from build123d import *

# Parameters (mm, degrees)
EXTRUDE_1_DEPTH     = 10
SKETCH_2_R          = 1.5
CUT_EXTRUDE_1_DEPTH = 10
CUT_EXTRUDE_2_REACH = 25.452
SKETCH_3_R          = 2


with BuildPart() as part:
    # 草图1 → 凸台-拉伸1 (new, symmetric)
    with BuildSketch(Plane.XY):
        Polygon((7.5, 0), (-7.5, 0), (-7.5, 15), (-15, 15), (-15, -5), (15, -5), (15, 15), (7.5, 15), align=None)
    extrude(amount=EXTRUDE_1_DEPTH, both=True)

    # 草图2 → 切除-拉伸1 (cut)
    with BuildSketch(Plane(origin=(0, 15, 0), x_dir=(1, 0, 0), z_dir=(0, 1, 0))):
        with Locations(Location((-11.1, 5, 0), (0, 0, 180))):
            Circle(SKETCH_2_R)
        with Locations(Location((11.1, -5, 0), (0, 0, 180))):
            Circle(SKETCH_2_R)
        with Locations((11.1, 5)):
            Circle(SKETCH_2_R)
        with Locations((-11.1, -5)):
            Circle(SKETCH_2_R)
    extrude(amount=-CUT_EXTRUDE_1_DEPTH, mode=Mode.SUBTRACT)

    # 草图3 → 切除-拉伸2 (cut, up to next)
    with BuildSketch(Plane(origin=(0, 0, 0), x_dir=(1, 0, 0), z_dir=(0, 1, 0)), mode=Mode.PRIVATE) as cut_extrude_2_sk1:
        with Locations(Location((0, 0, 0), (0, 0, 180))):
            Circle(SKETCH_3_R)
    cut_extrude_2_tool1 = extrude(cut_extrude_2_sk1.sketch, amount=-CUT_EXTRUDE_2_REACH, mode=Mode.PRIVATE) & part.part
    add(cut_extrude_2_tool1.solids().sort_by_distance((0, 0, 0))[0], mode=Mode.SUBTRACT)


solid = part.part
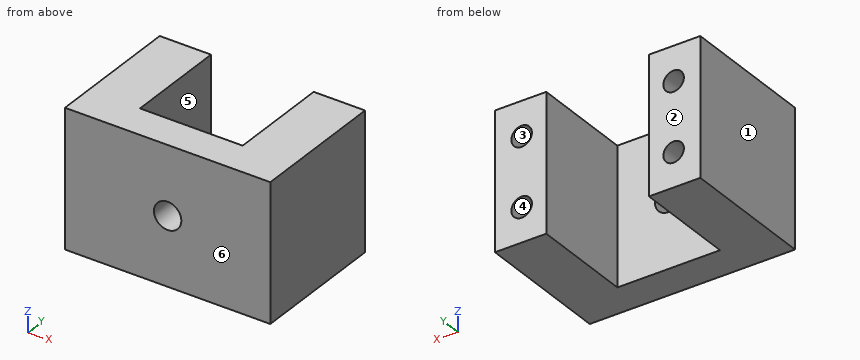
Work out the finished part from the listing and answer in its coordinate system (mm). Face numbers are marked on the shaded views. A direction names the side the tool comes from. Round coordinates to 2 decimals unless told otherwise and drop trailing zeros. Loops run counter-clockwise (first coordinate to the right, second up) from the corner with the lowest first, then second, coordinate; pieces in that order, holes last. Notation, with made-up numbers: (14.25, -35.75) - (27.25, -35.75) arc R32 ccw to (27.25, -9.75) - close; hole circle Ø6 at (60.25, 66.25). An arc over 180 degrees is marked (long way). Use one line per item in the form item = value. Start each with the question number.
(1) Find section A-A on y = 6.25. Determine the outline of the cut face in (x, z), and give its area (3 significant figures).
(2) Consider line 1 (Z direction, x = -11.1, y = 8.25); line 2 (Z direction, x = 0, y = -2.2); line 3 (X direction, y = 6.5, z = 2). Determine where each line is inside the solid, lowest interval first.
(3) Find section D-D on z = 5. Determine the outline of the cut face in (x, y), and give its area (3 significant figures).
(4) Determine the mould class of the marked faces 1, 2 and 3 for opening direction X: +X half, -X half, draft (parallel to the pull), parting line (faces both ways), or undercut.
(5) Find section C-C on x = 0. Determine the outline of the cut face in (y, z), and give its area (3 significant figures).
(6) Which of the six approach directions +Z, -Z, +X, -X, +Y, -Y give full straight-line access (tool end or side, diameter ignored) to the marked faces 4, 5 and 6?
(7) Flat-ended cylindrical pins translate along their axes: P1, Ø1.5, axis at x = 10.5, z = -5, coming from the +Y side; P2, Ø4, axis at x = 1.5, z = 0, coming from the +Y side; P3, Ø12, axis at x = -1, y = 11.5, coming from the +Z side. Find the tip coordinate at first contact, or state that the pin passes through.
(8) Find section B-B on z = 0. Determine the outline of the cut face in (x, y).
Answer list:
q1.outline = (-15, -10) - (-7.5, -10) - (-7.5, 10) - (-15, 10) - close; (7.5, -10) - (15, -10) - (15, 10) - (7.5, 10) - close; hole circle Ø3 at (-11.1, -5); hole circle Ø3 at (-11.1, 5); hole circle Ø3 at (11.1, -5); hole circle Ø3 at (11.1, 5)
q1.area = 272 mm^2
q2.line_1 = -10 to -6.5, -3.5 to 3.5, 6.5 to 10
q2.line_2 = -10 to -2, 2 to 10
q2.line_3 = -15 to -7.5, 7.5 to 15
q3.outline = (-15, -5) - (15, -5) - (15, 15) - (12.6, 15) - (12.6, 5) - (9.6, 5) - (9.6, 15) - (7.5, 15) - (7.5, 0) - (-7.5, 0) - (-7.5, 15) - (-9.6, 15) - (-9.6, 5) - (-12.6, 5) - (-12.6, 15) - (-15, 15) - close
q3.area = 315 mm^2
q4.face_1 = -X half
q4.face_2 = draft
q4.face_3 = undercut
q5.outline = (-5, -10) - (0, -10) - (0, -2) - (-5, -2) - close; (-5, 2) - (0, 2) - (0, 10) - (-5, 10) - close
q5.area = 80.0 mm^2
q6.face_4 = +Y
q6.face_5 = +Z, -Z, +Y
q6.face_6 = +Z, -Z, +X, -X, -Y
q7.P1 = 5
q7.P2 = 0
q7.P3 = through
q8.outline = (-15, -5) - (-2, -5) - (-2, 0) - (-7.5, 0) - (-7.5, 15) - (-15, 15) - close; (2, -5) - (15, -5) - (15, 15) - (7.5, 15) - (7.5, 0) - (2, 0) - close
